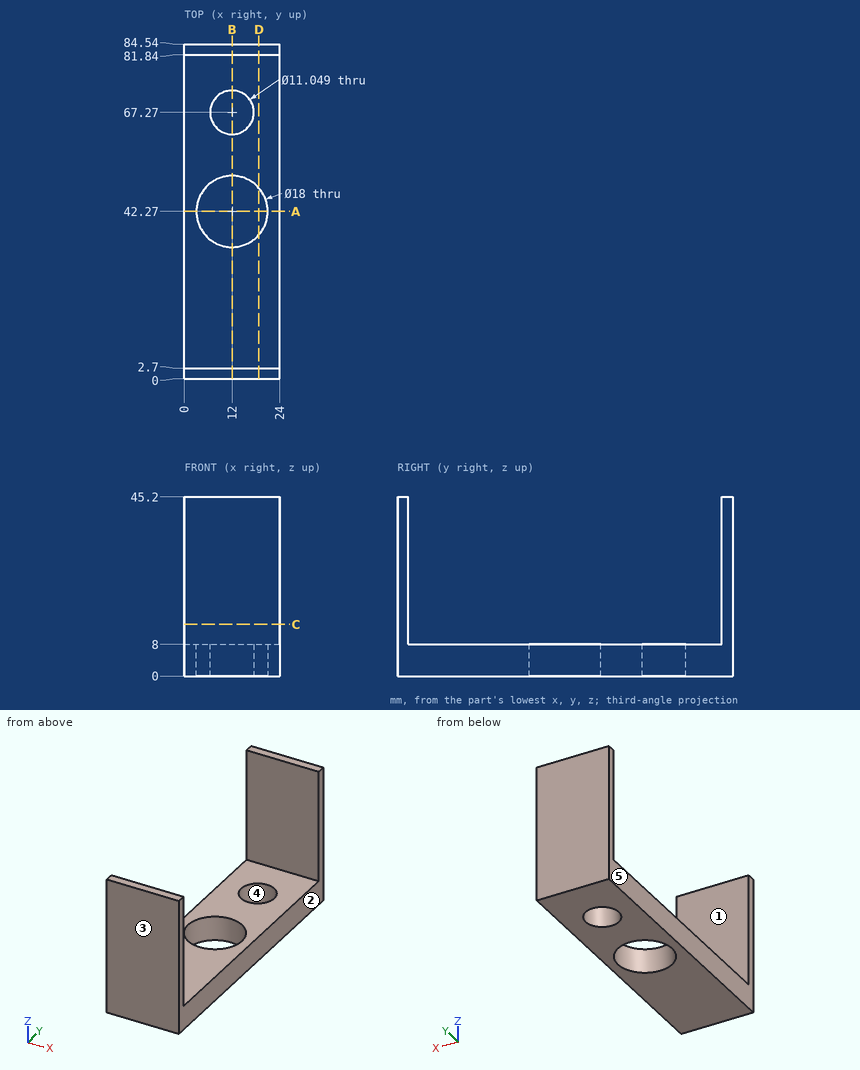
Answer from the drawing. Dimensions are ordinates in mm from the lowest x, y and z of the part. A direction names the side the tool comes from. Round coordinates to 2 decimals unless told otherwise and drop trailing zeros. Loops run counter-clockwise (first coordinate to the right, second up) from the corner with the lowest first, then second, coordinate; pieces in that order, holes last. Notation, with made-up numbers: M 45.25,64 L 64.25,64 A16 cw 64.25,85 Z; hole C -19.75,74.25 d11. An arc over 180 degrees is marked long. One line per question, with ' | ' between items. Start each with the question number.
(1) Find the intervals of material crossed by line 1 (Y direction, x = 12, z = 5.5); line 2 (X direction, y = 67, z = 3); line 3 (Y direction, x = 5.25, z = 31), in increasing order.
(2) A cutting plane is placed at A-A on y = 42.27. Write down the section's boundary in (x, z).
(3) A cutting plane is placed at D-D on x = 18.75. Write down the section's boundary in (y, z).
(4) For a pull along Y with two mould halves and no side action, classify the marked faces 3, 4 and 5 as released by +Y, released by -Y, zero draft, split by the parting line, or undercut.
(5) A cutting plane is placed at B-B on x = 12. Write down the section's boundary in (y, z).
(6) A tool of negligible diameter and unlimited length cuts with its end or side. For the marked faces 1 and 2, from which of +Z, -Z, +X, -X, +Y, -Y can it reach the whole face along a straight path? Write none if from no direction.
(7) A cutting plane is placed at C-C on z = 13. Write down the section's boundary in (x, y), plus the area to 3 significant figures.
(8) A flat-ended cylindrical pin translates along its axis: pin 1 Ø7 at (x, y) = (10, 55) entering from +Z. Find the tip coordinate at first contact, or state that the pin passes through.
Geometry check:
1) line 1: y = 0 to 33.27, 51.27 to 61.75, 72.79 to 84.54 | line 2: x = 0 to 6.48, 17.52 to 24 | line 3: y = 0 to 2.7, 81.84 to 84.54
2) outline: M 0,0 L 3,0 L 3,8 L 0,8 Z; M 21,0 L 24,0 L 24,8 L 21,8 Z
3) outline: M 0,0 L 36.32,0 L 36.32,8 L 2.7,8 L 2.7,45.2 L 0,45.2 Z; M 48.22,0 L 84.54,0 L 84.54,45.2 L 81.84,45.2 L 81.84,8 L 48.22,8 Z
4) face 3: released by -Y | face 4: undercut | face 5: zero draft
5) outline: M 0,0 L 33.27,0 L 33.27,8 L 2.7,8 L 2.7,45.2 L 0,45.2 Z; M 51.27,0 L 61.75,0 L 61.75,8 L 51.27,8 Z; M 72.79,0 L 84.54,0 L 84.54,45.2 L 81.84,45.2 L 81.84,8 L 72.79,8 Z
6) face 1: +Z, +X, -X | face 2: +Z, -Z, +X, +Y, -Y
7) outline: M 0,0 L 24,0 L 24,2.7 L 0,2.7 Z; M 0,81.84 L 24,81.84 L 24,84.54 L 0,84.54 Z | area: 130 mm²
8) pin 1: stops at z = 8
